```python
from build123d import *

# Parameters (mm, degrees)
SKETCH_1_W          = 16
SKETCH_1_H          = 10
EXTRUDE_1_DEPTH     = 3
SKETCH_2_R          = 2
CUT_EXTRUDE_1_DEPTH = 5


with BuildPart() as part:
    # 스케치1 → 보스-돌출1 (new, symmetric)
    with BuildSketch(Plane.XY):
        Rectangle(SKETCH_1_W, SKETCH_1_H)
    extrude(amount=EXTRUDE_1_DEPTH, both=True)

    # 스케치2 → 컷-돌출1 (cut)
    with BuildSketch(Plane.XZ.offset(5)):
        with Locations(Location((0, 0, 0), (0, 0, 270))):
            Circle(SKETCH_2_R)
    extrude(amount=-CUT_EXTRUDE_1_DEPTH, mode=Mode.SUBTRACT)


solid = part.part
```
Geometry check sheet. Reference: the model listing, model coordinates, mm. A direction names the side the tool comes from. Round coordinates to 2 decimals unless told otherwise and drop trailing zeros. Loops run counter-clockwise (first coordinate to the right, second up) from the corner with the lowest first, then second, coordinate; pieces in that order, holes last. Notation, with made-up numbers: M 4.5,88 L 10.5,88 A18 ccw 10.5,100 Z; hole C -19,-32.75 d6. An arc over 180 degrees is marked long. Return JSON: item names as keys, results as strings. Group by question number.
(1) Set-up check for faces 4 (the face through (-2, -3, 0)), 5 (the face through (0, 5, 0)): record each of +Z, -Z, +X, -X, +Y, -Y from which the full face is reachable in a straight line by a thin tool's end or side.
(2) Mould release check, pull along Z, two halves, no side actions. Record for faces 1 (the face through (0, 0, 0)), 2 (the face through (-8, 0, 0)), 3 (the face through (0, 0, -3)): pulls with the +Z half, pulls with the -Z half, needs draft (parallel to the pull), parting line crosses it, or undercut.
(3) Scan lines: line 1 along X through (y, z) = (-1.9, 0); line 2 along X through (y, z) = (-2.5, -0.5). Record each from-to range of solid material in increasing order. Write a range as [from, to].
(4) Section check C-C, the plane y = -1.75. Enter the section's corners in (x, z).
(5) Section check B-B, the plane x = 0. Enter the section's corners in (y, z).
(6) Section check A-A, the plane z = 0. Enter the section's corners in (x, y).
Data:
{
 "1": {"face 4": "-Y", "face 5": "+Z, -Z, +X, -X, +Y"},
 "2": {"face 1": "undercut", "face 2": "needs draft", "face 3": "pulls with the -Z half"},
 "3": {"line 1": "[-8, -2], [2, 8]", "line 2": "[-8, -1.94], [1.94, 8]"},
 "4": {"outline": "M -8,-3 L 8,-3 L 8,3 L -8,3 Z; hole C 0,0 d4"},
 "5": {"outline": "M -5,-3 L 5,-3 L 5,3 L -5,3 L -5,2 L 0,2 L 0,-2 L -5,-2 Z"},
 "6": {"outline": "M -8,-5 L -2,-5 L -2,0 L 2,0 L 2,-5 L 8,-5 L 8,5 L -8,5 Z"}
}
